```python
from build123d import *

# Parameters (mm, degrees)
BOSS_EXTRUDE1_DEPTH = 4
BOSS_EXTRUDE2_DEPTH = 40
SKETCH3_W           = 9
SKETCH3_H           = 16
BOSS_EXTRUDE3_DEPTH = 1
CHAMFER1_SIZE       = 1
SKETCH4_R           = 5.1
CUT_EXTRUDE1_DEPTH  = 31.25
CUT_EXTRUDE2_REACH  = 58.789
SKETCH5_R           = 2.55
FILLET1_R           = 1
SKETCH6_R           = 1.6
CUT_EXTRUDE3_DEPTH  = 56.794265031
SKETCH7_W           = 3
SKETCH7_H           = 3.5
CUT_EXTRUDE4_DEPTH  = 1.5
CHAMFER2_SIZE       = 1
SKETCH8_W           = 3.5
SKETCH8_H           = 9.5
CUT_EXTRUDE5_DEPTH  = 2
CHAMFER3_SIZE       = 1.5


with BuildPart() as part:
    # Sketch1 → Boss-Extrude1 (new body)
    with BuildSketch(Plane(origin=(0, 0, 0), x_dir=(1, 0, 0), z_dir=(0, 1, 0))):
        with BuildLine():
            Line((1, 0), (39, 0))
            ThreePointArc((39, 0), (39.707106781, 0.292893219), (40, 1))
            Line((40, 1), (40, 36))
            Line((40, 36), (0, 36))
            Line((0, 36), (0, 1))
            ThreePointArc((0, 1), (0.292893219, 0.292893219), (1, 0))
        make_face()
    extrude(amount=BOSS_EXTRUDE1_DEPTH)

    # Sketch2 → Boss-Extrude2 (add, through all)
    with BuildSketch(Plane(origin=(40, 0, 0), x_dir=(0, 0, -1), z_dir=(1, 0, 0))):
        with BuildLine():
            Line((36, 0), (36, 16))
            Line((36, 16), (31.25, 16))
            ThreePointArc((31.25, 16), (27.735281374, 7.514718626), (19.25, 4))
            Line((19.25, 4), (19.25, 0))
            Line((19.25, 0), (36, 0))
        make_face()
    extrude(amount=-BOSS_EXTRUDE2_DEPTH)

    # Sketch3 → Boss-Extrude3 (add)
    with BuildSketch(Plane(origin=(0, 0, -36), x_dir=(-1, 0, 0), z_dir=(0, 0, -1))):
        with Locations((-30, 8)):
            Rectangle(SKETCH3_W, SKETCH3_H)
        with Locations((-10, 8)):
            Rectangle(SKETCH3_W, SKETCH3_H)
    extrude(amount=BOSS_EXTRUDE3_DEPTH)

    # Chamfer1
    chamfer1_edges = [part.edges().sort_by_distance(p)[0] for p in [
        (25.5, 8, -37),
        (34.5, 8, -37),
        (14.5, 8, -37),
        (5.5, 8, -37),
    ]]
    chamfer(chamfer1_edges, length=CHAMFER1_SIZE - 0.0001)  # a hair under: the kernel refuses the full size

    # Sketch4 → Cut-Extrude1 (cut)
    with BuildSketch(Plane.XY):
        with Locations((10, 10)):
            Circle(SKETCH4_R)
        with Locations((30, 10)):
            Circle(SKETCH4_R)
    extrude(amount=-CUT_EXTRUDE1_DEPTH, mode=Mode.SUBTRACT)

    # Sketch5 → Cut-Extrude2 (cut, up to next)
    with BuildSketch(Plane(origin=(0, 0, -37), x_dir=(-1, 0, 0), z_dir=(0, 0, -1)), mode=Mode.PRIVATE) as cut_extrude2_sk1:
        with Locations((-30, 10)):
            Circle(SKETCH5_R)
    cut_extrude2_tool1 = extrude(cut_extrude2_sk1.sketch, amount=-CUT_EXTRUDE2_REACH, mode=Mode.PRIVATE) & part.part
    # Sketch5 → Cut-Extrude2 (cut, up to next)
    with BuildSketch(Plane(origin=(0, 0, -37), x_dir=(-1, 0, 0), z_dir=(0, 0, -1)), mode=Mode.PRIVATE) as cut_extrude2_sk2:
        with Locations((-10, 10)):
            Circle(SKETCH5_R)
    cut_extrude2_tool2 = extrude(cut_extrude2_sk2.sketch, amount=-CUT_EXTRUDE2_REACH, mode=Mode.PRIVATE) & part.part
    add(cut_extrude2_tool1.solids().sort_by_distance((30, 10, -37))[0], mode=Mode.SUBTRACT)
    add(cut_extrude2_tool2.solids().sort_by_distance((10, 10, -37))[0], mode=Mode.SUBTRACT)

    # Fillet1
    fillet1_edges = [part.edges().sort_by_distance(p)[0] for p in [
        (0, 16, -33.625),
        (40, 16, -33.625),
    ]]
    fillet(fillet1_edges, radius=FILLET1_R)

    # Sketch6 → Cut-Extrude3 (cut, through all)
    with BuildSketch(Plane(origin=(0, 4, 0), x_dir=(1, 0, 0), z_dir=(0, 1, 0))):
        with Locations(Location((36.4, 3.2, 0), (0, 0, 270))):
            Circle(SKETCH6_R)
        with Locations(Location((17.4, 3.2, 0), (0, 0, 270))):
            Circle(SKETCH6_R)
    extrude(amount=-CUT_EXTRUDE3_DEPTH, mode=Mode.SUBTRACT)

    # Sketch7 → Cut-Extrude4 (cut)
    with BuildSketch(Plane.XZ):
        with Locations((31.5, -9.5)):
            Rectangle(SKETCH7_W, SKETCH7_H)
        with Locations((26.75, -9.5)):
            Rectangle(SKETCH7_W, SKETCH7_H)
        with Locations((22, -9.5)):
            Rectangle(SKETCH7_W, SKETCH7_H)
    extrude(amount=-CUT_EXTRUDE4_DEPTH, mode=Mode.SUBTRACT)

    # Chamfer2
    chamfer2_edges = [part.edges().sort_by_distance(p)[0] for p in [
        (33, 1.5, -9.5),
        (30, 1.5, -9.5),
        (28.25, 1.5, -9.5),
        (25.25, 1.5, -9.5),
        (23.5, 1.5, -9.5),
        (20.5, 1.5, -9.5),
    ]]
    chamfer(chamfer2_edges, length=CHAMFER2_SIZE)

    # Sketch8 → Cut-Extrude5 (cut)
    with BuildSketch(Plane.XZ):
        with Locations((11.25, -8.5)):
            Rectangle(SKETCH8_W, SKETCH8_H)
    extrude(amount=-CUT_EXTRUDE5_DEPTH, mode=Mode.SUBTRACT)

    # Chamfer3
    chamfer3_edges = [part.edges().sort_by_distance(p)[0] for p in [
        (9.5, 2, -8.5),
        (13, 2, -8.5),
    ]]
    chamfer(chamfer3_edges, length=CHAMFER3_SIZE)


solid = part.part
```
Could you check a few things on this model? Use its own coordinates, in mm. A direction names the side the tool comes from. Round coordinates to 2 decimals unless told otherwise and drop trailing zeros. Loops run counter-clockwise (first coordinate to the right, second up) from the corner with the lowest first, then second, coordinate; pieces in that order, holes last.
Q1. I want a section at A-A (z = -33). Write out the boundary of the cut face in (x, y), and give its area (3 significant figures).
Q2. I want a section at C-C (z = -3.2). Write out the boundary of the cut face in (x, y), and give its area (3 significant figures).
Q3. For P1, Ø0.5, axis at x = 22, z = -10, coming from the -Y side; P2, Ø21, axis at x = 18, z = -8.5, coming from the +Y side; P3, Ø5.5, axis at x = 20, y = 6.5, coming from the -Z side, each with a flat end and sliding along its axis, tell me the tip position at first contact or that it passes through.
Q4. Thinking about a two-plate mould opening in Z: for faces 1 (the flat face through (27, 1, -11.25)), 2 (the cylindrical face through (0.285, 15.699, -33.571)), 3 (the flat face through (12, 8, -31.25)), which applies, pulls with the +Z half, pulls with the -Z half, needs draft (parallel to the pull), parting line crosses it, or undercut?
Q5. On a 3-axis mill with a long thin cutter (end or side, diameter ignored), from which of +Z, -Z, +X, -X, +Y, -Y can I reach the whole of each face in a straight line? I mean faces 4 (the flat face through (20, 0, -19)), 5 (the flat face through (22, 1, -7.75)), 6 (the flat face through (32, 8, -31.25)). Say none if no direction works.
Q6. I want a section at D-D (y = 10). Give the number of separate pieces and of enclosed holes in the cut face, and give its area (3 significant figures).
Q7. I want a section at B-B (x = 36.4). Write out the boundary of the cut face in (y, z).
Q8. Please list where these lines run through material, in increasing order: L1, parallel to X at y = 1.85, z = -3.2; L2, parallel to Y at x = 26.5, z = -19.5; L3, parallel to X at y = 3.5, z = -4.5.
Answer below:
1. outline: (0, 0) - (40, 0) - (40, 15) arc R1 ccw to (39, 16) - (1, 16) arc R1 ccw to (0, 15) - close; hole circle Ø5.1 at (10, 10); hole circle Ø5.1 at (30, 10)
1. area: 599 mm2
2. outline: (0, 0) - (15.8, 0) - (15.8, 4) - (0, 4) - close; (19, 0) - (34.8, 0) - (34.8, 4) - (19, 4) - close; (38, 0) - (40, 0) - (40, 4) - (38, 4) - close
2. area: 134 mm2
3. P1: stops at y = 1.5
3. P2: stops at y = 4
3. P3: stops at z = -36
4. face 1: undercut
4. face 2: needs draft
4. face 3: pulls with the +Z half
5. face 4: +Z, -Z, +X, -X, -Y
5. face 5: -Y
5. face 6: +Z
6. separate pieces: 3
6. enclosed holes: 0
6. area: 179 mm2
7. outline: (0, -36) - (16, -36) - (16, -31.25) arc R12 cw to (4, -19.25) - (4, -4.8) - (0, -4.8) - close; (0, -1.6) - (4, -1.6) - (4, 0) - (0, 0) - close
8. L1: x = 0 to 15.8, 19 to 34.8, 38 to 40
8. L2: y = 0 to 4
8. L3: x = 0 to 16.47, 18.33 to 35.47, 37.33 to 40
